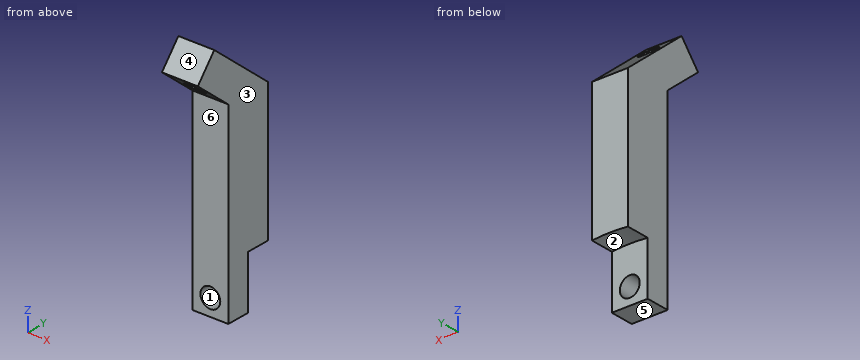
```python
from build123d import *

# Parameters (mm, degrees)
SKETCH1_W           = 15
SKETCH1_H           = 80
SKETCH1_R           = 4.15
BOSS_EXTRUDE1_DEPTH = 10
BOSS_EXTRUDE2_DEPTH = 10
BOSS_EXTRUDE4_DEPTH = 15
SKETCH11_R          = 4
CUT_EXTRUDE5_DEPTH  = 31.247894791


with BuildPart() as part:
    # Sketch1 → Boss-Extrude1 (new body)
    with BuildSketch(Plane(origin=(0, 0, 0), x_dir=(1, 0, 0), z_dir=(0, 1, 0))):
        Rectangle(SKETCH1_W, SKETCH1_H)
        with Locations((0, 33)):
            Circle(SKETCH1_R, mode=Mode.SUBTRACT)
    extrude(amount=BOSS_EXTRUDE1_DEPTH)

    # Sketch2 → Boss-Extrude2 (add)
    with BuildSketch(Plane(origin=(0, 10, 0), x_dir=(1, 0, 0), z_dir=(0, 1, 0))):
        with BuildLine():
            Line((7.5, 17.775942217), (7.5, -40))
            Line((7.5, -40), (-7.5, -40))
            Line((-7.5, -40), (-7.5, 17.775942217))
            ThreePointArc((-7.5, 17.775942217), (0, 17.4), (7.5, 17.775942217))
        make_face()
    extrude(amount=BOSS_EXTRUDE2_DEPTH)

    # Sketch10 → Boss-Extrude4 (add)
    with BuildSketch(Plane(origin=(7.5, 0, 0), x_dir=(0, 0, -1), z_dir=(1, 0, 0))):
        Polygon((-40, 0), (-52.855752194, -15.320888862), (-62.703829724, -7.057370639), (-40, 20), align=None)
    extrude(amount=-BOSS_EXTRUDE4_DEPTH)

    # Sketch11 → Cut-Extrude5 (cut, through all)
    with BuildSketch(Plane(origin=(0, 19.69615506, 23.472963553), x_dir=(-1, 0, 0), z_dir=(0, -0.64278761, -0.766044443))):
        with Locations((0, -35.711504387)):
            Circle(SKETCH11_R)
    extrude(amount=-CUT_EXTRUDE5_DEPTH, mode=Mode.SUBTRACT)


solid = part.part
```
Model file for the job. Use its own axes, mm. Face numbers are marked on the shaded views. A direction names the side the tool comes from. Coordinates: 2 decimals unless noted, no trailing zeros. Loops run counter-clockwise (first coordinate to the right, second up) from the corner with the lowest first, then second, coordinate; pieces in that order, holes last. Notation, with made-up numbers: (21, -35.5) - (70, -35.5) arc R30 cw to (70, 3.5) - close; hole circle Ø3 at (46.25, 56). An arc over 180 degrees is marked (long way). Write item = value, one per line. Start each with the question number.
Item 1: Wall check: probe 1 along X at (y, z) = (3, -33); probe 2 along Y at (x, z) = (3, -25); probe 3 along Y at (x, z) = (3.5, -17). Give the ranges that are in metal, low to high. Write a range as [from, to].
Item 2: Saw through at A-A, the plane z = -33. List the corners of the cut face in (x, y), then the cut area to 3 significant figures.
Item 3: Saw through at D-D, the plane z = 19. List the corners of the cut face in (x, y), then the cut area to 3 significant figures.
Item 4: Saw through at C-C, the plane y = 9. List the corners of the cut face in (x, z).
Item 5: 3-axis set-ups, long thin cutter, end or side, ignore diameter. For the marked faces 5 and 6: which of +Z, -Z, +X, -X, +Y, -Y reach the whole face in a straight line?
Item 6: Drop flat-ended pins along their axis: pin 1 Ø1.5 at (x, y) = (-4.5, 3) entering from +Z; pin 2 Ø6 at (x, y) = (-1.5, -5.5) entering from -Z; pin 3 Ø2 at (x, z) = (5.5, 3) entering from -Y; pin 4 Ø6.5 at (x, z) = (0, -33) entering from -Y. Give the stop position or say it passes through.
Item 7: Saw through at B-B, the plane x = 0. List the corners of the cut face in (y, z).
Item 8: Pull direction X, two halves, no side cores. Call the marked faces 1, 2, 3 and 4: +X half, -X half, draft (parallel to the pull), parting line (faces both ways), or undercut.
Answers:
q1.probe_1 = [-7.5, -4.15], [4.15, 7.5]
q1.probe_2 = [0, 10]
q1.probe_3 = [0, 20]
q2.outline = (-7.5, 0) - (-4.15, 0) - (-4.15, 10) - (-7.5, 10) - close; (4.15, 0) - (7.5, 0) - (7.5, 10) - (4.15, 10) - close
q2.area = 67.0 mm2
q3.outline = (-7.5, 0) - (7.5, 0) - (7.5, 20) - (-7.5, 20) - close
q3.area = 300 mm2
q4.outline = (-7.5, -40) - (7.5, -40) - (7.5, 49.23) - (-7.5, 49.23) - close; hole circle Ø8.3 at (0, -33)
q5.face_5 = -Z, +X, -X, +Y, -Y
q5.face_6 = -Z, +X, -X, -Y
q6.pin_1 = 54.89
q6.pin_2 = 42.1
q6.pin_3 = 0
q6.pin_4 = through
q7.outline = (-15.32, 52.86) - (-10.72, 49) - (-2.46, 58.85) - (-7.06, 62.7) - close; (-4.6, 43.86) - (0, 40) - (0, -28.85) - (10, -28.85) - (10, -17.4) - (20, -17.4) - (20, 40) - (3.67, 53.7) - close; (0, -40) - (10, -40) - (10, -37.15) - (0, -37.15) - close
q8.face_1 = undercut
q8.face_2 = undercut
q8.face_3 = +X half
q8.face_4 = draft
